For this review, take the finished solid that the model builds, in its own axes (mm). A direction names the side the tool comes from. Round coordinates to 2 decimals unless told otherwise and drop trailing zeros. Write each loop counter-clockwise with the first axis right and the second up, starting at its lowest first coordinate (ties: lowest second). Pieces come first, ordered by that corner, then holes. Notation, with made-up numbers: (53.25, 38) - (104.25, 38) arc R13 cw to (104.25, 44) - close; hole circle Ø10 at (-36, 10.5). An arc over 180 degrees is marked (long way). One line per item, written item: value. Start each with the question number.
Q1. Add section B-B on y = 9.5. Give the number of separate pieces and of enclosed holes in the cut face, and give its area (3 significant figures).
Q2. Add section D-D on z = 16. Write out the cut boundary in (x, y).
Q3. Add section A-A on x = 0. Write out the cut boundary in (y, z), and give its area (3 significant figures).
Q4. For probe 1 along Z at (x, y) = (0, 2.5); probe 2 along Y at (x, z) = (1, 12.5); probe 3 along X at (y, z) = (2, 24), list the stretches that pass through material, from the lowest coordinate up.
Q5. Tool access review of faces 5 (the face through (-17.54, 9.57, -18.03)), 6 (the face through (17.54, 9.57, 18.03)), 7 (the face through (-12.817, 9.481, 22.047)), 8 (the face through (-13.791, 9.569, 14.245)): name each direction out of +Z, -Z, +X, -X, +Y, -Y from which nothing blocks a thin tool from reaching the whole face with its end or side.
Q6. Mouldability with a two-part tool opening along Z and no side actions: class faces 1 (the face through (0, 3, 31.75)), 2 (the face through (-6.842, 9.569, -24.204)), 3 (the face through (13.815, 9.569, 14.246)), 4 (the face through (-9.802, 9.481, -16.865)) as +Z half, -Z half, draft (parallel to the pull), parting line (faces both ways), or undercut.
Q7. Clearance check with a flat-ended pin moving along its axis: pin 1 Ø6 at (x, z) = (11.5, -2.5) entering from +Y. State where the tip first meets the part, or that it passes through.
Q8. Add section C-C on z = 0. Write out the cut boundary in (x, y), and give its area (3 significant figures).
```python
from build123d import *

# Parameters (mm, degrees)
SKETCH1_W                 = 38.1
SKETCH1_H                 = 63.5
BOSS_EXTRUDE1_DEPTH       = 6.35
BOSS_EXTRUDE2_DEPTH       = 6.35
FILLET1_R                 = 1.143
CIRPATTERN1_COUNT         = 6
FILLET1_OF_CIRPATTERN1_R  = 1.143
SKETCH3_R                 = 8.89
CUT_EXTRUDE1_DEPTH        = 7.35
F_8_32_TAPPED_HOLE1_D     = 3.4544
F_8_32_TAPPED_HOLE1_DEPTH = 6.35


with BuildPart() as part:
    # Sketch1 → Boss-Extrude1 (new body)
    with BuildSketch(Plane(origin=(0, 0, 0), x_dir=(1, 0, 0), z_dir=(0, 1, 0))):
        Rectangle(SKETCH1_W, SKETCH1_H)
    extrude(amount=BOSS_EXTRUDE1_DEPTH)

    # Sketch2 → Boss-Extrude2 (add)
    with BuildSketch(Plane(origin=(0, 6.35, 0), x_dir=(1, 0, 0), z_dir=(0, 1, 0))):
        with BuildLine():
            Line((-18.032354291, 18.032354291), (-13.793673402, 13.793673402))
            ThreePointArc((-13.793673402, 13.793673402), (-9.7536, 16.893730757), (-5.048834877, 18.842508279))
            Line((-5.048834877, 18.842508279), (-6.600299761, 24.632654052))
            ThreePointArc((-6.600299761, 24.632654052), (-12.7508, 22.085033437), (-18.032354291, 18.032354291))
        make_face()
    boss_extrude2 = extrude(amount=BOSS_EXTRUDE2_DEPTH)

    # Fillet1
    fillet1_edges = [part.edges().sort_by_distance(p)[0] for p in [
        (-6.600299761, 9.525, -24.632654052),
        (-18.032354291, 9.525, -18.032354291),
        (-13.793673402, 9.525, -13.793673402),
        (-5.048834877, 9.525, -18.842508279),
    ]]
    fillet(fillet1_edges, radius=FILLET1_R)

    # CirPattern1: Boss-Extrude2 ×6 about axis, 2 skipped
    cirpattern1_axis = Axis((0, 12.7, 0), (0, 1, 0))
    add([boss_extrude2.rotate(cirpattern1_axis, i * 360 / CIRPATTERN1_COUNT) for i in range(1, CIRPATTERN1_COUNT) if i not in (1, 4)])

    # Fillet1 of CirPattern1
    fillet1_of_cirpattern1_edges = [part.edges().sort_by_distance(p)[0] for p in [
        (-18.032354291, 9.525, 18.032354291),
        (-6.600299761, 9.525, 24.632654052),
        (-5.048834877, 9.525, 18.842508279),
        (-13.793673402, 9.525, 13.793673402),
        (6.600299761, 9.525, 24.632654052),
        (18.032354291, 9.525, 18.032354291),
        (13.793673402, 9.525, 13.793673402),
        (5.048834877, 9.525, 18.842508279),
        (18.032354291, 9.525, -18.032354291),
        (6.600299761, 9.525, -24.632654052),
        (5.048834877, 9.525, -18.842508279),
        (13.793673402, 9.525, -13.793673402),
    ]]
    fillet(fillet1_of_cirpattern1_edges, radius=FILLET1_OF_CIRPATTERN1_R)

    # Sketch3 → Cut-Extrude1 (cut, through all)
    with BuildSketch(Plane(origin=(0, 6.35, 0), x_dir=(1, 0, 0), z_dir=(0, 1, 0))):
        Circle(SKETCH3_R)
    extrude(amount=-CUT_EXTRUDE1_DEPTH, mode=Mode.SUBTRACT)

    # #8-32 Tapped Hole1
    with Locations(Plane(origin=(0, 6.35, 0), x_dir=(1, 0, 0), z_dir=(0, 1, 0))):
        with Locations((0, -23.8125), (0, 23.8125)):
            Hole(F_8_32_TAPPED_HOLE1_D / 2, depth=F_8_32_TAPPED_HOLE1_DEPTH)


solid = part.part
```
Result set:
1. separate pieces: 4
1. enclosed holes: 0
1. area: 278 mm^2
2. outline: (-19.05, 0) - (19.05, 0) - (19.05, 6.35) - (16, 6.35) - (16, 12.7) - (11.16, 12.7) - (11.16, 6.35) - (-11.16, 6.35) - (-11.16, 12.7) - (-16, 12.7) - (-16, 6.35) - (-19.05, 6.35) - close
3. outline: (0, -31.75) - (6.35, -31.75) - (6.35, -25.54) - (0, -25.54) - close; (0, -22.09) - (6.35, -22.09) - (6.35, -8.89) - (0, -8.89) - close; (0, 8.89) - (6.35, 8.89) - (6.35, 22.09) - (0, 22.09) - close; (0, 25.54) - (6.35, 25.54) - (6.35, 31.75) - (0, 31.75) - close
3. area: 246 mm^2
4. probe 1: z = -31.75 to -25.54, -22.09 to -8.89, 8.89 to 22.09, 25.54 to 31.75
4. probe 2: y = 0 to 6.35
4. probe 3: x = -19.05 to -1.72, 1.72 to 19.05
5. face 5: -X, +Y
5. face 6: +X, +Y
5. face 7: +Z, -X, +Y
5. face 8: +Y
6. face 1: +Z half
6. face 2: -Z half
6. face 3: undercut
6. face 4: undercut
7. pin 1: stops at y = 6.35
8. outline: (-19.05, 0) - (-8.89, 0) - (-8.89, 6.35) - (-19.05, 6.35) - close; (8.89, 0) - (19.05, 0) - (19.05, 6.35) - (8.89, 6.35) - close
8. area: 129 mm^2
